from build123d import *

# Parameters (mm, degrees)
SKETCH1_R           = 53
BOSS_EXTRUDE1_DEPTH = 78
SKETCH2_R           = 10
BOSS_EXTRUDE2_DEPTH = 26
SKETCH9_R           = 17.4625
BOSS_EXTRUDE4_DEPTH = 4.25
SKETCH12_W          = 137.4
SKETCH12_H          = 72
BOSS_EXTRUDE6_DEPTH = 24
SKETCH13_R          = 2
CUT_EXTRUDE2_DEPTH  = 24


with BuildPart() as part:
    # Sketch1 → Boss-Extrude1 (new, symmetric)
    with BuildSketch(Plane(origin=(0, 0, 0), x_dir=(1, 0, 0), z_dir=(0, 1, 0))):
        with Locations(Location((0, 0, 0), (0, 0, 270))):
            Circle(SKETCH1_R)
    extrude(amount=BOSS_EXTRUDE1_DEPTH, both=True)

    # Sketch2 → Boss-Extrude2 (add)
    with BuildSketch(Plane(origin=(0, 78, 0), x_dir=(1, 0, 0), z_dir=(0, 1, 0))):
        with Locations(Location((0, 0, 0), (0, 0, 90))):
            Circle(SKETCH2_R)
    extrude(amount=BOSS_EXTRUDE2_DEPTH)

    # Sketch9 → Boss-Extrude4 (add, symmetric)
    with BuildSketch(Plane(origin=(0, 97, 0), x_dir=(1, 0, 0), z_dir=(0, 1, 0))):
        with Locations(Location((0, 0, 0), (0, 0, 270))):
            Circle(SKETCH9_R)
    extrude(amount=BOSS_EXTRUDE4_DEPTH, both=True)

    # Sketch12 → Boss-Extrude6 (add)
    with BuildSketch(Plane(origin=(0, 0, 69), x_dir=(-1, 0, 0), z_dir=(0, 0, -1))):
        Rectangle(SKETCH12_W, SKETCH12_H)
    extrude(amount=BOSS_EXTRUDE6_DEPTH)

    # Sketch13 → Cut-Extrude2 (cut)
    with BuildSketch(Plane.XY.offset(69)):
        with Locations((-58.7, -26)):
            Circle(SKETCH13_R)
        with Locations((-58.7, 26)):
            Circle(SKETCH13_R)
        with Locations((58.7, 26)):
            Circle(SKETCH13_R)
        with Locations((58.7, -26)):
            Circle(SKETCH13_R)
    extrude(amount=-CUT_EXTRUDE2_DEPTH, mode=Mode.SUBTRACT)


solid = part.part
Can you work these out from the model? Positions are in its coordinate system, mm. A direction names the side the tool comes from. Round coordinates to 2 decimals unless told otherwise and drop trailing zeros. Write each loop counter-clockwise with the first axis right and the second up, starting at its lowest first coordinate (ties: lowest second). Pieces come first, ordered by that corner, then holes. Notation, with made-up numbers: M 41.5,87 L 63.5,87 A34 cw 63.5,122 Z; hole C -30.5,2.25 d1. An arc over 180 degrees is marked long. Use a Markdown table: item, result.
Item 1: I want a section at B-B (x = 0). List the corners of the cut face in (y, z) for me, and give its area (3 significant figures).
Found:
| item | result |
|---|---|
| outline | M -78,-53 L 78,-53 L 78,-10 L 92.75,-10 L 92.75,-17.46 L 101.25,-17.46 L 101.25,-10 L 104,-10 L 104,10 L 101.25,10 L 101.25,17.46 L 92.75,17.46 L 92.75,10 L 78,10 L 78,53 L 36,53 L 36,69 L -36,69 L -36,53 L -78,53 Z |
| area | 18,300 mm2 |
Item 2: Which directions (+Z, -Z, +X, -X, +Y, -Y) give clear straight access to the entire face, cutting with the end or side of a thin tool? Please do faces 1 (the face through (-8, 92.75, 8)), 2 (the face through (1, 36, 57)), 3 (the face through (-8, 101.25, 8)), 4 (the face through (1, -36, 57)).
Found:
| item | result |
|---|---|
| face 1 | none |
| face 2 | +Z, +Y |
| face 3 | +Y |
| face 4 | +Z, -Y |
Item 3: I want a section at D-D (x = 38.5). List the corners of the cut face in (y, z) for me, and give its area (3 significant figures).
Found:
| item | result |
|---|---|
| outline | M -78,-36.42 L 78,-36.42 L 78,36.42 L -78,36.42 Z; M -36,45 L 36,45 L 36,69 L -36,69 Z |
| area | 13,100 mm2 |
Item 4: For pin 1 Ø12 at (x, y) = (-40.5, 14.5) entering from -Z; pin 2 Ø8 at (x, y) = (-36, 25) entering from -Z; pin 3 Ø6 at (y, z) = (38.5, 41.5) entering from +X, each with a flat end and sliding along its axis, tell me the tip position at first contact or that it passes through.
Found:
| item | result |
|---|---|
| pin 1 | stops at z = -40.23 |
| pin 2 | stops at z = -42.25 |
| pin 3 | stops at x = 36.42 |
Item 5: We'd pull the mould along X, two halves only. Please class faces 5 (the face through (0, 104, 0)), 6 (the face through (56.702, -25.912, 57.168)), 7 (the face through (9.76, 85.27, 2.17)): released by +X, released by -X, zero draft, split by the parting line, or undercut.
Found:
| item | result |
|---|---|
| face 5 | zero draft |
| face 6 | undercut |
| face 7 | split by the parting line |
Item 6: I want a section at C-C (y = -20). List the corners of the cut face in (x, z) for me, and give its area (3 significant figures).
Found:
| item | result |
|---|---|
| outline | M -68.7,45 L -28,45 A53 ccw long 28,45 L 68.7,45 L 68.7,69 L -68.7,69 Z |
| area | 11,800 mm2 |
Item 7: If I drill on line 1 along Y through (x, z) = (58.7, 56); line 2 along Y through (x, z) = (58, 52); line 3 along Z through (x, y) = (-1, 30.5), over which ranges is the centre line in solid material (lowest first)? Write a range as [from, to].
Found:
| item | result |
|---|---|
| line 1 | y = [-36, -28], [-24, 24], [28, 36] |
| line 2 | y = [-36, -27.87], [-24.13, 24.13], [27.87, 36] |
| line 3 | z = [-52.99, 69] |
Item 8: I want a section at A-A (z = 0). List the corners of the cut face in (x, y) for me, and give its area (3 significant figures).
Found:
| item | result |
|---|---|
| outline | M -53,-78 L 53,-78 L 53,78 L 10,78 L 10,92.75 L 17.46,92.75 L 17.46,101.25 L 10,101.25 L 10,104 L -10,104 L -10,101.25 L -17.46,101.25 L -17.46,92.75 L -10,92.75 L -10,78 L -53,78 Z |
| area | 17,200 mm2 |
